```python
from build123d import *

# Parameters (mm, degrees)
BOSS_EXTRUDE1_DEPTH = 36
BOSS_EXTRUDE3_DEPTH = 10
SKETCH4_R           = 0.5
BOSS_EXTRUDE4_DEPTH = 2


with BuildPart() as part:
    # Sketch1 → Boss-Extrude1 (new body)
    with BuildSketch(Plane.XY):
        Polygon((63.072235962, 55.72786335), (64.072235962, 55.72786335), (66.572235962, 20.72786335), (60.572235962, 20.72786335), align=None)
    extrude(amount=-BOSS_EXTRUDE1_DEPTH)

    # Sketch3 → Boss-Extrude3 (add)
    with BuildSketch(Plane.XY):
        Polygon((60.572235962, 20.72786335), (60.929378819, 25.72786335), (66.215093105, 25.72786335), (66.572235962, 20.72786335), align=None)
    extrude(amount=BOSS_EXTRUDE3_DEPTH)

    # Sketch4 → Boss-Extrude4 (add)
    with BuildSketch(Plane.XY.offset(10)):
        Polygon((66.572235962, 20.72786335), (60.572235962, 20.72786335), (62.072235962, 2.52786335), (65.072235962, 2.52786335), align=None)
        with Locations(Location((63.572235962, 14.52786335, 0), (0, 0, 180))):
            Circle(SKETCH4_R, mode=Mode.SUBTRACT)
        with Locations(Location((63.572235962, 12.52786335, 0), (0, 0, 180))):
            Circle(SKETCH4_R, mode=Mode.SUBTRACT)
        with Locations(Location((63.572235962, 10.52786335, 0), (0, 0, 180))):
            Circle(SKETCH4_R, mode=Mode.SUBTRACT)
        with Locations(Location((63.572235962, 8.52786335, 0), (0, 0, 180))):
            Circle(SKETCH4_R, mode=Mode.SUBTRACT)
        with Locations(Location((63.572235962, 4.52786335, 0), (0, 0, 180))):
            Circle(SKETCH4_R, mode=Mode.SUBTRACT)
        with Locations(Location((63.572235962, 6.52786335, 0), (0, 0, 180))):
            Circle(SKETCH4_R, mode=Mode.SUBTRACT)
    extrude(amount=-BOSS_EXTRUDE4_DEPTH)


solid = part.part
```
Work out the finished part from the listing and answer in its coordinate system (mm). A direction names the side the tool comes from. Give positions to 0.01 mm unless a question says otherwise; leave off trailing zeros. Write each loop counter-clockwise with the first axis right and the second up, starting at its lowest first coordinate (ties: lowest second). Pieces come first, ordered by that corner, then holes. Notation, with made-up numbers: (20.5, -9.5) -> (64.5, -9.5) arc R7 ccw to (64.5, -5.5) -> close; hole circle Ø1 at (-17.5, 45.25). An arc over 180 degrees is marked (long way). Write each question's results on one line, items separated by ' | '.
1. Find section B-B on y = 28. Determine the outline of the cut face in (x, z), and give its area (3 significant figures).
Data:
outline: (61.09, -36) -> (66.05, -36) -> (66.05, 0) -> (61.09, 0) -> close | area: 179 mm^2
2. A tool of negligible diameter and unlimited length cuts with its end or side. For faces 1 (the flat face through (64, 38, 0)), 2 (the flat face through (65.81, 11.5, 9.01)), 3 (the flat face through (64, 14, 8)), from which of +Z, -Z, +X, -X, +Y, -Y can it reach the whole face along a straight path? Write none if from no direction.
Data:
face 1: +Z, +X, -X, +Y | face 2: +Z, -Z, +X, -Y | face 3: -Z, +X, -X, -Y
3. Each of these flat-tipped pins is pushed along its axis until it touches: pin 1 Ø1.6 at (x, z) = (62.5, 3.5) entering from +Y; pin 2 Ø3 at (x, y) = (63, 8.5) entering from -Z; pin 3 Ø1.5 at (x, z) = (64.5, -23) entering from -Y. Where does it stop, or does it pass through?
Data:
pin 1: y = 25.73 | pin 2: z = 8 | pin 3: y = 20.73
4. Find section A-A on z = -28. Determine the outline of the cut face in (x, y).
Data:
outline: (60.57, 20.73) -> (66.57, 20.73) -> (64.07, 55.73) -> (63.07, 55.73) -> close
5. Straight lines are drawn through the part: L1, parallel to Y at x = 65.4, z = 3.5; L2, parallel to Z at x = 65.65, y = 14; L3, parallel to Y at x = 63.8, z = -24. For each, find the intervals that lie inside material, in ascending order.
Data:
L1: 20.73 to 25.73 | L2: 8 to 10 | L3: 20.73 to 55.73
